Here's the drawing with two shaded views (mm, measured from the low corner). I have some questions. A direction names the side the tool comes from. Give positions to 0.01 mm unless a question says otherwise; leave off trailing zeros. Loops run counter-clockwise (first coordinate to the right, second up) from the corner with the lowest first, then second, coordinate; pieces in that order, holes last. Notation, with made-up numbers: (3, 32) -> (23, 32) arc R24 ccw to (23, 57) -> close; hole circle Ø5 at (57.5, -10). An arc over 180 degrees is marked (long way). Put each result on its own line as item: value.
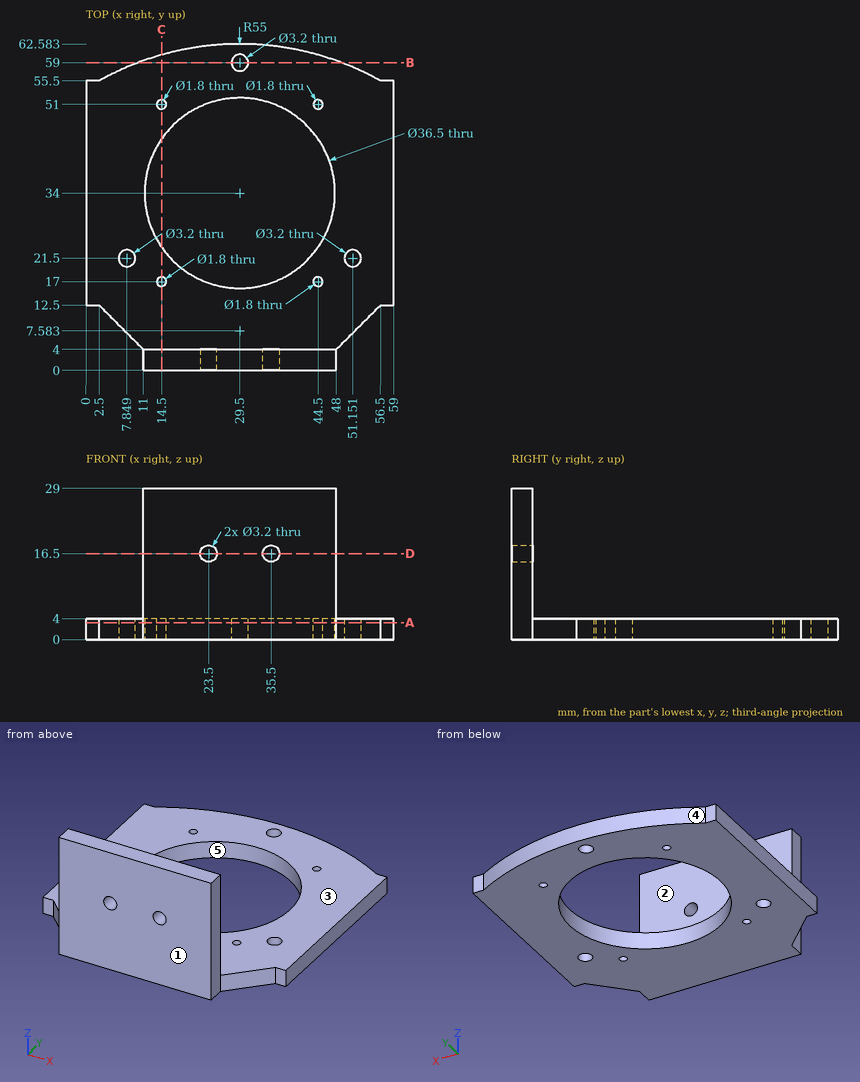
1. If we section it at C-C (x = 14.5): List the corners of the cut face in (y, z) for me (1 decimal).
Recorded:
outline: (0, 0) -> (16.1, 0) -> (16.1, 4) -> (4, 4) -> (4, 29) -> (0, 29) -> close; (17.9, 0) -> (23.6, 0) -> (23.6, 4) -> (17.9, 4) -> close; (44.4, 0) -> (50.1, 0) -> (50.1, 4) -> (44.4, 4) -> close; (51.9, 0) -> (60.5, 0) -> (60.5, 4) -> (51.9, 4) -> close
2. If we section it at D-D (z = 16.5): List the corners of the cut face in (x, y) for me, then the cut area to 3 significant figures.
Recorded:
outline: (11, 0) -> (21.9, 0) -> (21.9, 4) -> (11, 4) -> close; (25.1, 0) -> (33.9, 0) -> (33.9, 4) -> (25.1, 4) -> close; (37.1, 0) -> (48, 0) -> (48, 4) -> (37.1, 4) -> close
area: 122 mm^2
3. If we section it at A-A (z = 3.25): Count the separate pieces of the cut face and the enclosed holes in it, then the cut area to 3 significant figures.
Recorded:
separate pieces: 1
enclosed holes: 8
area: 2,250 mm^2
4. I need wall thicknesses on line 1 (Y direction, x = 29.5, z = 1.3); line 2 (Z direction, x = 35.5, y = 3.2); line 3 (Y direction, x = 44.5, z = 2.5) (1 decimal). Which ranges of each line are inside material? Lowest first, please.
Recorded:
line 1: y = 0 to 15.75, 52.25 to 57.4, 60.6 to 62.58
line 2: z = 0 to 14.9, 18.1 to 29
line 3: y = 0 to 16.1, 17.9 to 23.6, 44.4 to 50.1, 51.9 to 60.5
5. If we section it at B-B (y = 59): List the corners of the cut face in (x, z) for me.
Recorded:
outline: (9.97, 0) -> (27.9, 0) -> (27.9, 4) -> (9.97, 4) -> close; (31.1, 0) -> (49.03, 0) -> (49.03, 4) -> (31.1, 4) -> close
6. I'm going to push flat-ended pins straight in: pin 1 (4.5 mm diameter, centred on y = 1.5, z = 18.5, fed in from +X); pin 2 (1.2 mm diameter, centred on x = 1, z = 3, fed in from -Y); pin 3 (0.8 mm diameter, centred on x = 1, z = 3, fed in from +Y). Where does each tip first touch, or does it pass through?
Recorded:
pin 1: stops at x = 48
pin 2: stops at y = 12.5
pin 3: stops at y = 55.5
7. For the marked faces 1 and 2, which set-ups out of +Z, -Z, +X, -X, +Y, -Y let a thin tool reach every point of the face, with its end or its side?
Recorded:
face 1: +Z, -Z, +X, -X, -Y
face 2: +Z, +X, -X, +Y
8. Thinking about a two-plate mould opening in X: for the marked faces 3, 4 and 5, which applies, pulls with the +X half, pulls with the -X half, needs draft (parallel to the pull), parting line crosses it, or undercut?
Recorded:
face 3: needs draft
face 4: parting line crosses it
face 5: undercut
